Autodesk Inventor part; units mm, degrees
ref_plane "Start Plane" through (0, 0, 0) normal (1, 0, 0) x (0, 1, 0)
ref_plane "XZ Plane" through (0, 0, 0) normal (0, 1, 0) x (-1, 0, 0)
ref_plane "XY Plane" through (0, 0, 0) normal (0, 0, 1) x (1, 0, 0)
sketch "Main Sketch" plane through (0, 0, 0) normal (0, 0, 1) x (1, 0, 0)
  line L0 (0, 0) -> (180, 0)
  line L1 (0, 0) -> (0, 15)
  line L2 (0, 15) -> (40, 15)
  line L3 (40, 15) -> (40, 20)
  line L4 (90, 20) -> (90, 15)
  line L5 (40, 20) -> (90, 20)
  line L6 (90, 15) -> (100, 15)
  line L7 (100, 15) -> (100, 17.5)
  line L8 (140, 17.5) -> (140, 15)
  line L9 (100, 17.5) -> (140, 17.5)
  line L10 (180, 15) -> (180, 0)
  line L11 (140, 15) -> (180, 15)
  dimension "d3" = 30
  dimension "d4" = 40
  dimension "d5" = 30
  dimension "d6" = 35
  dimension "d7" = 30
revolve "Revolution1" add sketch "Main Sketch" angle 360 about axis through (0, 0, 0) along (1, 0, 0)
chamfer "Chamfer1" distance 2 angle 45 1 edges at (40, -15, 0) measured on face at (26.6667, 14.8058, -2.4062)
chamfer "Chamfer2" distance 2 angle 45 1 edges at (90, -15, 0) measured on face at (96.6667, 14.8058, -2.4062)
chamfer "Chamfer3" distance 2 angle 45 1 edges at (100, -15, 0) measured on face at (97.3333, 14.9514, -1.207)
chamfer "Chamfer4" distance 2 angle 45 1 edges at (140, -15, 0) measured on face at (166.6667, 14.8058, -2.4062)
equation "\"Length\" = 180"
properties part number "Shaft" material "Steel"
Can you work these out from the model? Positions are in its coordinate system, mm. A direction names the side the tool comes from. Coordinates: 2 decimals unless noted, no trailing zeros. Write each loop counter-clockwise with the first axis right and the second up, starting at its lowest first coordinate (ties: lowest second). Pieces come first, ordered by that corner, then holes.
Q1. Imagine slicing it at C-C, the plane x = 60. List the corners of the cut face in (y, z) for me, plus the area to 3 significant figures.
Results found:
outline: circle Ø40 at (0, 0)
area: 1,260 mm2
Q2. Imagine slicing it at D-D, the plane x = 21.5. List the corners of the cut face in (y, z) for me, plus the area to 3 significant figures.
Results found:
outline: circle Ø30 at (0, 0)
area: 707 mm2
Q3. Which directions (+Z, -Z, +X, -X, +Y, -Y) give clear straight access to the entire face, cutting with the end or side of a thin tool? Please do faces 4 (the face through (40, -9, -15)), 5 (the face through (100, -3, 17)), 6 (the face through (140, -3, 17)), 7 (the face through (65.35, -4.336, -19.524)).
Results found:
face 4: -X
face 5: none
face 6: +X
face 7: +X, -X
Q4. For P1, Ø1.5, axis at x = 123.5, z = 13, coming from the +Y side; P2, Ø5, axis at x = 77.5, y = -11, coming from the -Z side; P3, Ø12, axis at x = 153, z = 3, coming from the -Y side, each with a flat end and sliding along its axis, tell me the tip position at first contact or that it passes through.
Results found:
P1: stops at y = 12.5
P2: stops at z = -18.1
P3: stops at y = -15
Q5. Imagine slicing it at A-A, the plane y = 0. List the corners of the cut face in (x, z) for me.
Results found:
outline: (0, -15) - (38, -15) - (40, -17) - (40, -20) - (90, -20) - (90, -17) - (92, -15) - (98, -15) - (100, -17) - (100, -17.5) - (140, -17.5) - (140, -17) - (142, -15) - (180, -15) - (180, 15) - (142, 15) - (140, 17) - (140, 17.5) - (100, 17.5) - (100, 17) - (98, 15) - (92, 15) - (90, 17) - (90, 20) - (40, 20) - (40, 17) - (38, 15) - (0, 15) - close
Q6. Please list where these lines run through material, in increasing order: L1, parallel to X at y = -5.5, z = 16.5; L2, parallel to X at y = 18, z = -5; L3, parallel to X at y = -8, z = -13.5.
Results found:
L1: x = 40 to 90, 100 to 140
L2: x = 40 to 90
L3: x = 38.69 to 91.31, 98.69 to 141.31
Q7. If we mould it in two halves opening along X, with no side actions, what happens to faces 1 (the face through (120.28, -13.887, -10.648)), 2 (the face through (180, 0, 0)), 3 (the face through (98.13, -3.28, -14.77))? For each: +X half, -X half, draft (parallel to the pull), parting line (faces both ways), or undercut.
Results found:
face 1: draft
face 2: +X half
face 3: undercut
